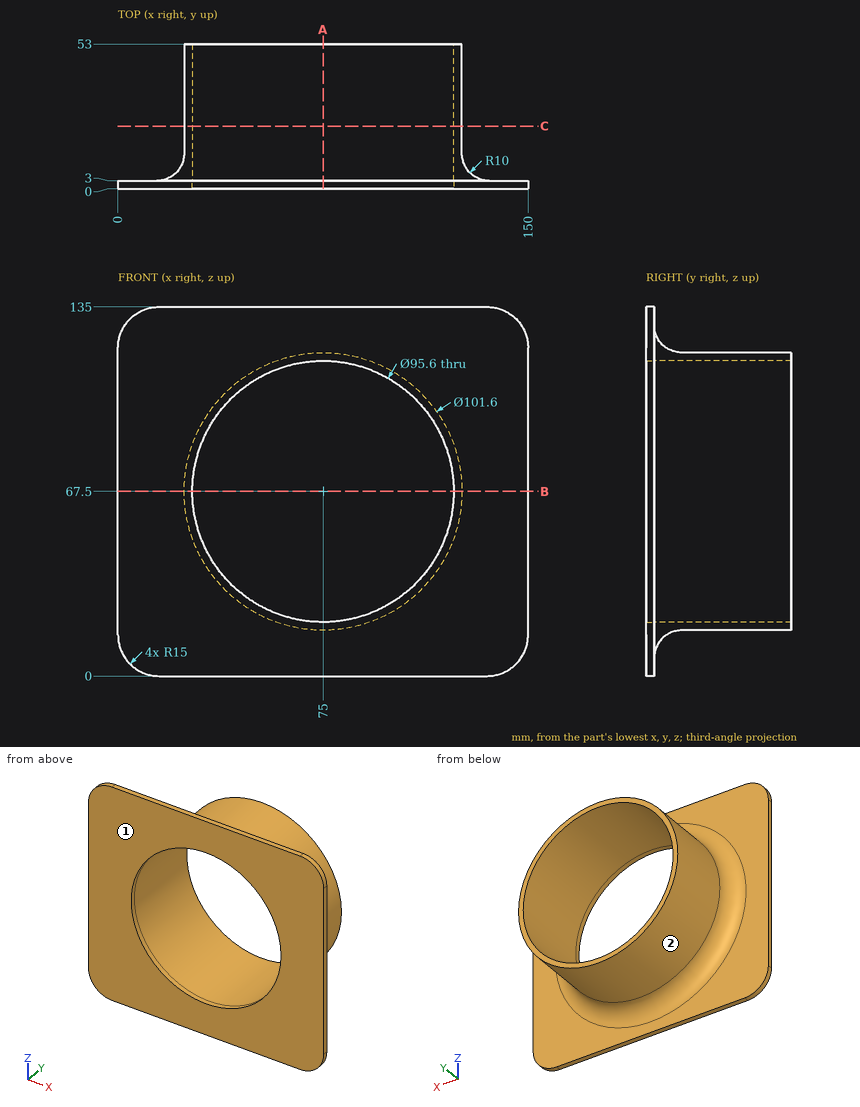
Job drawing, mm, ordinate dimensions from the low corner. One solid piece. A direction names the side the tool comes from. Give positions to 0.01 mm unless a question says otherwise; leave off trailing zeros. Order: outer loops, then holes, each group sorted by start corner. A loop starts at its lowest first (then second) coordinate and runs counter-clockwise, first axis right, second up. Notation, with made-up numbers: (88, 83.25) - (142, 83.25) arc R12 ccw to (142, 97.25) - close; hole circle Ø5 at (57, 51). An arc over 180 degrees is marked (long way). One line per question, with ' | ' between items.
1. Band-saw the part on B-B on z = 67.5. List the corners of the cut face in (x, y).
Filled in:
outline: (0, 0) - (27.2, 0) - (27.2, 53) - (24.2, 53) - (24.2, 13) arc R10 cw to (14.2, 3) - (0, 3) - close; (122.8, 0) - (150, 0) - (150, 3) - (135.8, 3) arc R10 cw to (125.8, 13) - (125.8, 53) - (122.8, 53) - close
2. Drop flat-ended pins along their axis: P1, Ø1.5, axis at y = 30, z = 98.5, coming from the +X side; P2, Ø10, axis at x = 53.5, z = 13.5, coming from the -Y side; P3, Ø5, axis at x = 124.5, y = 19.5, coming from the +Z side; P4, Ø8, axis at y = 30, z = 97, coming from the +X side. Give the stop position or say it passes through.
Filled in:
P1: x = 115.81 | P2: y = 0 | P3: z = 86.78 | P4: x = 118.94
3. Drill centre lines: probe 1 along X at (y, z) = (29, 67.5); probe 2 along Z at (x, y) = (75, 2.15); probe 3 along Z at (x, y) = (75, 38.5). Where is each one in solid material? Low to high.
Filled in:
probe 1: 24.2 to 27.2, 122.8 to 125.8 | probe 2: 0 to 19.7, 115.3 to 135 | probe 3: 16.7 to 19.7, 115.3 to 118.3
4. Band-saw the part on A-A on x = 75. List the corners of the cut face in (y, z), then the cut area to 3 significant figures.
Filled in:
outline: (0, 0) - (3, 0) - (3, 6.7) arc R10 cw to (13, 16.7) - (53, 16.7) - (53, 19.7) - (0, 19.7) - close; (0, 115.3) - (53, 115.3) - (53, 118.3) - (13, 118.3) arc R10 cw to (3, 128.3) - (3, 135) - (0, 135) - close | area: 461 mm²
5. Which spindle directions (+Z, -Z, +X, -X, +Y, -Y) get a long thin tool onto all of the face, cutting with end or side? Do the marked faces 1 and 2. Say none if no direction does.
Filled in:
face 1: +Z, -Z, +X, -X, -Y | face 2: +Y
6. Band-saw the part on C-C on y = 23. List the corners of the cut face in (x, z).
Filled in:
outline: circle Ø101.6 at (75, 67.5); hole circle Ø95.6 at (75, 67.5)
